```python
from build123d import *

# Parameters (mm, degrees)
SKETCH4_W           = 9
SKETCH4_H           = 4
BOSS_EXTRUDE1_START = -1
SKETCH5_W           = 1.3
SKETCH5_H           = 5.75
BOSS_EXTRUDE1_DEPTH = 2.218926
SKETCH6_R           = 0.5
BOSS_EXTRUDE2_DEPTH = 3.5
SKETCH7_R           = 1.35
BOSS_EXTRUDE3_DEPTH = 2.5


with BuildPart() as part:
    # Sketch4 → Revolve3 (revolve)
    with BuildSketch(Plane.XY):
        with Locations((0, 2)):
            Rectangle(SKETCH4_W, SKETCH4_H)
    revolve(axis=Axis((-4.5, 4, 0), (1, 0, 0)))

    # Sketch5 → Boss-Extrude1 (add)
    with BuildSketch(Plane(origin=(0, 0, 0), x_dir=(1, 0, 0), z_dir=(0, 1, 0)).offset(BOSS_EXTRUDE1_START)):
        Rectangle(SKETCH5_W, SKETCH5_H)
    extrude(amount=BOSS_EXTRUDE1_DEPTH)

    # Sketch6 → Boss-Extrude2 (add)
    with BuildSketch(Plane(origin=(4.5, 0, 0), x_dir=(0, 0, -1), z_dir=(1, 0, 0))):
        with Locations((0, 4)):
            Circle(SKETCH6_R)
    extrude(amount=BOSS_EXTRUDE2_DEPTH)

    # Sketch7 → Boss-Extrude3 (add)
    with BuildSketch(Plane(origin=(8, 0, 0), x_dir=(0, 0, -1), z_dir=(1, 0, 0))):
        with Locations((0, 4)):
            Circle(SKETCH7_R)
    extrude(amount=-BOSS_EXTRUDE3_DEPTH)


solid = part.part
```
For this review, take the finished solid that the model builds, in its own axes (mm). A direction names the side the tool comes from. Round coordinates to 2 decimals unless told otherwise and drop trailing zeros. Write each loop counter-clockwise with the first axis right and the second up, starting at its lowest first coordinate (ties: lowest second). Pieces come first, ordered by that corner, then holes. Notation, with made-up numbers: (41, 34.25) - (48, 34.25) arc R22 cw to (48, 55.25) - close; hole circle Ø7 at (-6.5, 37). An arc over 180 degrees is marked (long way). Answer as a JSON object with one key per item and string values.
1. We need section B-B on y = 4. Give the boundary of the cut face in (x, z), then the cut area to 4 significant figures.
Response values:
{"outline": "(-4.5, -4) - (4.5, -4) - (4.5, -0.5) - (5.5, -0.5) - (5.5, -1.35) - (8, -1.35) - (8, 1.35) - (5.5, 1.35) - (5.5, 0.5) - (4.5, 0.5) - (4.5, 4) - (-4.5, 4) - close", "area": "79.75 mm2"}
2. We need section C-C on x = -3.5. Give the boundary of the cut face in (y, z).
Response values:
{"outline": "circle Ø8 at (4, 0)"}
3. Tool access review of faces 1 (the face through (0, -1, 0)), 2 (the face through (5.5, 4, -1)), 3 (the face through (0, 0, 2.875)), 4 (the face through (0, 0, -2.875)), 5 (the face through (6.77, 2.8, -0.62)): name each direction out of +Z, -Z, +X, -X, +Y, -Y from which nothing blocks a thin tool from reaching the whole face with its end or side.
Response values:
{"face 1": "+Z, -Z, +X, -X, -Y", "face 2": "none", "face 3": "+Z, +X, -X, -Y", "face 4": "-Z, +X, -X, -Y", "face 5": "+X"}
4. To check wall thickness, follow line 1 along X through (y, z) = (3, 0.5); line 2 along X through (y, z) = (4.5, 2.5); line 3 along X through (y, z) = (0.25, -2.25). State the ranges of each line that lie inside material, in increasing order.
Response values:
{"line 1": "x = -4.5 to 4.5, 5.5 to 8", "line 2": "x = -4.5 to 4.5", "line 3": "x = -0.65 to 0.65"}
5. We need section A-A on z = 0. Give the boundary of the cut face in (x, y).
Response values:
{"outline": "(-4.5, 0) - (-0.65, 0) - (-0.65, -1) - (0.65, -1) - (0.65, 0) - (4.5, 0) - (4.5, 3.5) - (5.5, 3.5) - (5.5, 2.65) - (8, 2.65) - (8, 5.35) - (5.5, 5.35) - (5.5, 4.5) - (4.5, 4.5) - (4.5, 8) - (-4.5, 8) - close"}
6. Draft analysis for pull direction X (two halves, no side actions). For faces 6 (the face through (0.65, -0.4, 0)), 7 (the face through (-0.65, -0.4, 0)), 8 (the face through (4.993, 4.496, 0.065)), state which applies: +X half, -X half, draft (parallel to the pull), parting line (faces both ways), or undercut.
Response values:
{"face 6": "+X half", "face 7": "-X half", "face 8": "undercut"}
7. For pin 1 Ø0.6 at (x, y) = (0.5, 0.5) entering from +Z (3 decimals); pin 2 Ø1.5 at (x, z) = (5, 3) entering from -Y; pin 3 Ø1.1 at (y, z) = (0, -1) entering from +X, all flat-tipped, find the tip position at first contact; note any pin that passes through.
Response values:
{"pin 1": "stops at z = 2.875", "pin 2": "stops at y = 0.83", "pin 3": "stops at x = 4.5"}
8. We need section D-D on z = 1.75. Give the boundary of the cut face in (x, y), then the cut area to 3 significant figures.
Response values:
{"outline": "(-4.5, 0.4) - (-0.65, 0.4) - (-0.65, -1) - (0.65, -1) - (0.65, 0.4) - (4.5, 0.4) - (4.5, 7.6) - (-4.5, 7.6) - close", "area": "66.6 mm2"}
